```python
from build123d import *

# Parameters (mm, degrees)
SKETCH4_W          = 0.866666667
SKETCH4_H          = 0.866666667
CHAMFER1_SIZE      = 0.26
CHAMFER2_SIZE      = 0.75
CHAMFER3_SIZE      = 0.4225
CUT_EXTRUDE1_DEPTH = 3
SKETCH15_R         = 4
CUT_EXTRUDE3_DEPTH = 2.825


with BuildPart() as part:
    # Sketch3 → Revolve1 (revolve)
    with BuildSketch(Plane(origin=(0, 0, 0), x_dir=(0, 0, -1), z_dir=(1, 0, 0))):
        Polygon((-31, 6.5), (-25, 6.5), (-25, 4), (20, 4), (20, 3), (31, 3), (31, 0), (-31, 0), align=None)
    revolve(axis=Axis((0, 0, -31), (0, 0, 1)))

    # Sketch4 → Cut-Revolve1 (revolve, cut)
    with BuildSketch(Plane(origin=(0, 0, 0), x_dir=(0, 0, -1), z_dir=(1, 0, 0))):
        with Locations((-24.566666667, 3.566666667)):
            Rectangle(SKETCH4_W, SKETCH4_H)
    revolve(axis=Axis((0, 0, -31), (0, 0, 1)), mode=Mode.SUBTRACT)

    # Chamfer1
    chamfer1_edges = [part.edges().sort_by_distance(p)[0] for p in [
        (0, -3.133333333, 24.133333333),
        (0, -4, 24.133333333),
    ]]
    chamfer(chamfer1_edges, length=CHAMFER1_SIZE)

    # Sketch6 → Cut-Revolve2 (revolve, cut)
    with BuildSketch(Plane(origin=(0, 0, 0), x_dir=(0, 0, -1), z_dir=(1, 0, 0))):
        with BuildLine():
            Line((20, 4), (24.4, 4))
            Line((24.4, 4), (22.6, 2.2))
            Line((22.6, 2.2), (20.8, 2.2))
            ThreePointArc((20.8, 2.2), (20.234314575, 2.434314575), (20, 3))
            Line((20, 3), (20, 4))
        make_face()
    revolve(axis=Axis((0, 0, -31), (0, 0, 1)), mode=Mode.SUBTRACT)

    # Chamfer2
    chamfer2_edges = [part.edges().sort_by_distance(p)[0] for p in [
        (0, -3, -31),
    ]]
    chamfer(chamfer2_edges, length=CHAMFER2_SIZE)

    # Chamfer3
    chamfer3_edges = [part.edges().sort_by_distance(p)[0] for p in [
        (0, -4, -20),
        (0, -6.5, 31),
    ]]
    chamfer(chamfer3_edges, length=CHAMFER3_SIZE)

    # Sketch8 → Cut-Extrude1 (cut)
    with BuildSketch(Plane.XY.offset(31)):
        Polygon((2, 1.154700538), (0, 2.309401077), (-2, 1.154700538), (-2, -1.154700538), (0, -2.309401077), (2, -1.154700538), align=None)
    extrude(amount=-CUT_EXTRUDE1_DEPTH, mode=Mode.SUBTRACT)

    # Cut-Extrude2 cone 1 section (through the dimple's axis) → Cut-Extrude2 (revolve, cut)
    with BuildSketch(Plane(origin=(0, 0, 31), x_dir=(0, -1, 0), z_dir=(1, 0, 0))):
        Polygon((0, 0), (2.309401077, 0), (0, 2.309401077), align=None)
    revolve(axis=Axis((0, 0, 31), (0, 0, -1)), mode=Mode.SUBTRACT)

    # Sketch15 → Cut-Extrude3 (cut)
    with BuildSketch(Plane(origin=(0, 0, -31), x_dir=(-1, 0, 0), z_dir=(0, 0, -1))):
        with Locations(Location((0, 0, 0), (0, 0, 90))):
            Circle(SKETCH15_R)
    extrude(amount=-CUT_EXTRUDE3_DEPTH, mode=Mode.SUBTRACT)


solid = part.part
```
Input: part model. Units: mm. Frame: model coordinates. A direction names the side the tool comes from. Round coordinates to 2 decimals unless told otherwise and drop trailing zeros. Loops run counter-clockwise (first coordinate to the right, second up) from the corner with the lowest first, then second, coordinate; pieces in that order, holes last. Notation, with made-up numbers: (17.25, 72) - (21.25, 72) arc R28 cw to (21.25, 99) - close; hole circle Ø5 at (5.25, 42). An arc over 180 degrees is marked (long way). One line per item, written item: value. Start each with the question number.
(1) Contact query for flat-ended pins moving along their axis: P1, Ø1, axis at x = 2.5, z = 18, coming from the +Y side; P2, Ø3, axis at y = 4.5, z = 9.5, coming from the +X side; P3, Ø2, axis at x = 2, z = -4.5, coming from the -Y side; P4, Ø1, axis at y = 5, z = -7.5, coming from the -X side. Output: stop coordinate, or through.
(2) Ray query, line 1 (Z direction, x = 1.75, y = -5); line 2 (X direction, y = -2.5, z = -9); line 3 (Z direction, x = -1.75, y = 1.25) (3 decimals). Return the intervals inside material, ascending. Write a range as [from, to].
(3) Section A-A, the plane z = -2. Return loops of the section in (x, y).
(4) Access query for faces 1 (the flat face through (0, 0, -28.175)), 2 (the cylindrical face through (3.905, -0.867, 1.844)), 3 (the conical face through (-1.06, -1.87, 30.84)). Directions: +Z, -Z, +X, -X, +Y, -Y. A direction counts if a zero-diameter tool reaches every point of the face in a straight line with its end or side. Return the directions, or none.
(5) Section B-B, the plane z = 27.5. Return loops of the section in (x, y), plus the area to 3 significant figures.
Results below:
1. P1: y = 3.46
1. P2: x = 2.65
1. P3: y = -3.87
1. P4: through
2. line 1: [25, 31]
2. line 2: [-3.12, 3.12]
2. line 3: [-28.175, 28]
3. outline: circle Ø8 at (0, 0)
4. face 1: -Z, +X, -X, +Y, -Y
4. face 2: -Z
4. face 3: +Z
5. outline: circle Ø13 at (0, 0)
5. area: 133 mm^2
